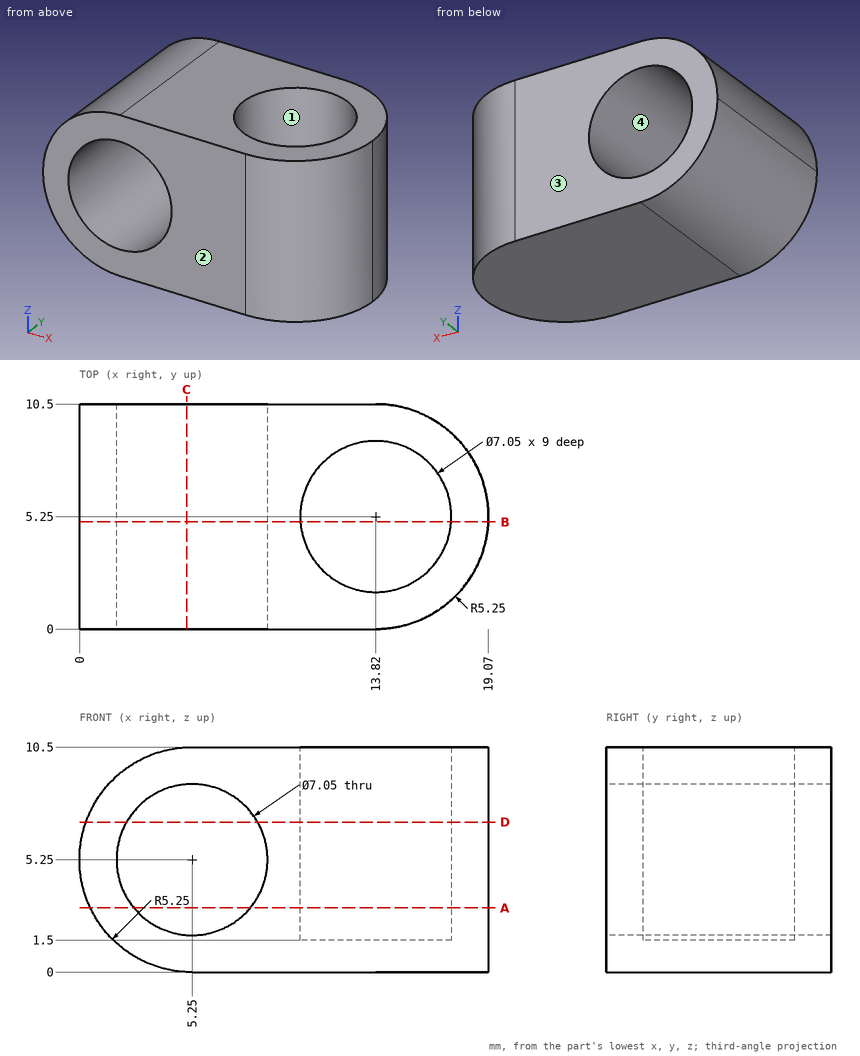
The figure shows three views and two pictorial views of one solid part (mm, origin at its lowest corner). Answer the questions. A direction names the side the tool comes from. Round coordinates to 2 decimals unless told otherwise and drop trailing zeros. Write each loop counter-clockwise with the first axis right and the second up, starting at its lowest first coordinate (ties: lowest second). Pieces come first, ordered by that corner, then holes. Notation, with made-up numbers: (0, 75) - (26, 75) arc R15 cw to (26, 86) - close; hole circle Ø6 at (66, -38). An arc over 180 degrees is marked (long way). Use one line per item in the form item = value. Start each with the question number.
Item 1: A cutting plane is placed at A-A (z = 3). Give the number of separate pieces and of enclosed holes in the cut face, plus the area to 3 significant figures.
Item 2: A cutting plane is placed at D-D (z = 7). Write down the section's boundary in (x, y) (3 decimals).
Item 3: A tool of negligible diameter and unlimited length cuts with its end or side. For the marked faces 1 and 2, from which of +Z, -Z, +X, -X, +Y, -Y can it reach the whole face along a straight path? Write none if from no direction.
Item 4: Determine the mould class of the marked faces 3 and 4 for opening direction X: +X half, -X half, draft (parallel to the pull), parting line (faces both ways), or undercut.
Item 5: A cutting plane is placed at B-B (y = 5). Write down the section's boundary in (x, z) (3 decimals), plus the area to 3 significant figures.
Item 6: A cutting plane is placed at C-C (x = 5). Write down the section's boundary in (y, z), plus the area to 3 significant figures.
Item 7: Flat-ended cylindrical pins translate along their axes: pin 1 Ø1 at (x, z) = (15, 1.5) entering from -Y; pin 2 Ø4 at (y, z) = (2.5, 5.5) entering from +X. Find the tip coordinate at first contact, or state that the pin passes through.
Item 8: Find the intervals of material crossed by line 1 (X direction, y = 4.75, z = 6.5); line 2 (Y direction, x = 14, z = 9.25); line 3 (Z direction, x = 16.5, y = 7), in increasing order. Write a range as [from, to].
The answers:
q1.separate_pieces = 2
q1.enclosed_holes = 1
q1.area = 87.1 mm^2
q2.outline = (0.3, 0) - (2.19, 0) - (2.19, 10.5) - (0.3, 10.5) - close; (8.31, 0) - (13.82, 0) arc R5.25 ccw to (19.07, 5.25) arc R5.25 ccw to (13.82, 10.5) - (8.31, 10.5) - close; hole circle Ø7.05 at (13.82, 5.25)
q3.face_1 = +Z
q3.face_2 = +Z, -Z, +X, -X, -Y
q4.face_3 = draft
q4.face_4 = undercut
q5.outline = (0, 5.25) arc R5.25 ccw to (5.25, 0) - (19.064, 0) - (19.064, 10.5) - (17.336, 10.5) - (17.336, 1.5) - (10.304, 1.5) - (10.304, 10.5) - (5.25, 10.5) arc R5.25 ccw to start; hole circle Ø7.05 at (5.25, 5.25)
q5.area = 86.0 mm^2
q6.outline = (0, 0.01) - (10.5, 0.01) - (10.5, 1.73) - (0, 1.73) - close; (0, 8.77) - (10.5, 8.77) - (10.5, 10.49) - (0, 10.49) - close
q6.area = 36.3 mm^2
q7.pin_1 = 0.04
q7.pin_2 = 19.02
q8.line_1 = [0.15, 1.95], [8.55, 10.33], [17.31, 19.05]
q8.line_2 = [0, 1.73], [8.77, 10.5]
q8.line_3 = [0, 1.5]
